Verification items for the finished model (mm, model axes). Give positions to 0.01 mm unless a question says otherwise; leave off trailing zeros. Write each loop counter-clockwise with the first axis right and the second up, starting at its lowest first coordinate (ties: lowest second). Pieces come first, ordered by that corner, then holes. Notation, with made-up numbers: M -15.5,72 L 8.5,72 A24 ccw 8.5,94 Z; hole C 66.25,-1.5 d11. An arc over 180 degrees is marked long. Write item = value, one per line.
from build123d import *

# Parameters (mm, degrees)
SKETCH1_W           = 186.616953842
SKETCH1_H           = 285.110155161
BOSS_EXTRUDE1_DEPTH = 1.5875
SKETCH2_R           = 11.15
CUT_EXTRUDE1_DEPTH  = 4.175


with BuildPart() as part:
    # Sketch1 → Boss-Extrude1 (new body, symmetric)
    with BuildSketch(Plane.XY):
        with Locations((93.308476921, 142.555077581)):
            Rectangle(SKETCH1_W, SKETCH1_H)
    extrude(amount=BOSS_EXTRUDE1_DEPTH, both=True)

    # Sketch2 → Cut-Extrude1 (cut, through all)
    with BuildSketch(Plane.XY.offset(1.5875)):
        with Locations((90.33901258, 97.817400981)):
            Circle(SKETCH2_R)
        with Locations((34.339946259, 97.494026403)):
            Circle(SKETCH2_R)
    extrude(amount=-CUT_EXTRUDE1_DEPTH, mode=Mode.SUBTRACT)


solid = part.part
1) Draft check along X on faces 1 (the cylindrical face through (31.92, 86.61, 0.02)), 2 (the flat face through (92, 145, 1.588)), 3 (the cylindrical face through (87.922, 86.933, 0.022)). Enter one of: +X half, -X half, draft (parallel to the pull), parting line (faces both ways), or undercut.
From the geometry:
face_1 = undercut
face_2 = draft
face_3 = undercut
2) Cross-section at A-A on y = 91.5. Record the boundary of the cut face in (x, z).
From the geometry:
outline = M 0,-1.59 L 24.94,-1.59 L 24.94,1.59 L 0,1.59 Z; M 43.74,-1.59 L 81.15,-1.59 L 81.15,1.59 L 43.74,1.59 Z; M 99.53,-1.59 L 186.62,-1.59 L 186.62,1.59 L 99.53,1.59 Z
3) Material ranges on probe 1 along Y at (x, z) = (36, -0.7); probe 2 along Y at (x, z) = (85.5, -0.95), recorded low to high. Write a range as from..to.
From the geometry:
probe_1 = 0..86.47, 108.52..285.11
probe_2 = 0..87.77, 107.86..285.11
